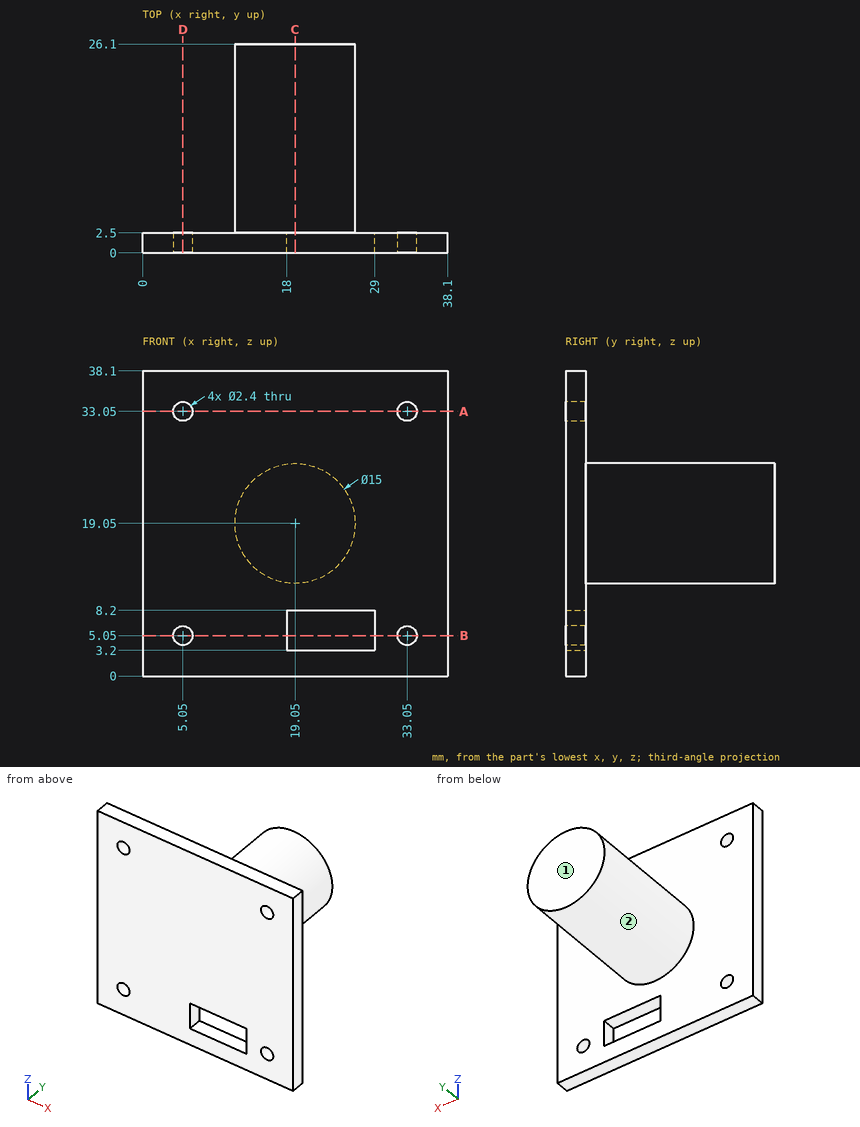
Could you check a few things on this drawing? It's one solid part, dimensions in mm from its lowest x, y, z. A direction names the side the tool comes from. Give positions to 0.01 mm unless a question says otherwise; leave off trailing zeros. Loops run counter-clockwise (first coordinate to the right, second up) from the corner with the lowest first, then second, coordinate; pieces in that order, holes last. Notation, with made-up numbers: (2, -14.75) -> (41, -14.75) arc R16 ccw to (41, 3.25) -> close; hole circle Ø5 at (77, 35). An arc over 180 degrees is marked (long way). Use one line per item in the form item = value. Start each with the question number.
1) For P1, Ø3, axis at x = 14.5, y = 18.5, coming from the +Z side; P2, Ø2, axis at x = 25, y = 1.5, coming from the -Z side; P3, Ø12, axis at y = 10, z = 26, coming from the +X side; P4, Ø1, axis at y = 11.5, z = 16, coming from the +X side, each with a flat end and sliding along its axis, tell me the tip position at first contact or that it passes through.
2) Which directions (+Z, -Z, +X, -X, +Y, -Y) give clear straight access to the entire face, cutting with the end or side of a thin tool? Please do the marked faces 1 and 2.
3) Imagine slicing it at B-B (z = 5.05). Please give me the cut outline in (x, y).
4) Imagine slicing it at C-C (x = 19.05). Please give me the cut outline in (y, z), then the cut area to 3 significant figures.
5) Imagine slicing it at A-A (z = 33.05). Please give me the cut outline in (x, y).
6) Imagine slicing it at D-D (x = 5.05). Please give me the cut outline in (y, z), then the cut area to 4 significant figures.
7) Please list where these lines run through material, in increasing order: line 1 along Z through (x, y) = (5.05, 1.45); line 2 along Y through (x, z) = (17, 9.5).
Check values:
q1.P1 = 25.9
q1.P2 = 0
q1.P3 = 26.49
q1.P4 = 26.1
q2.face_1 = +Z, -Z, +X, -X, +Y
q2.face_2 = +Y
q3.outline = (0, 0) -> (3.85, 0) -> (3.85, 2.5) -> (0, 2.5) -> close; (6.25, 0) -> (18, 0) -> (18, 2.5) -> (6.25, 2.5) -> close; (29, 0) -> (31.85, 0) -> (31.85, 2.5) -> (29, 2.5) -> close; (34.25, 0) -> (38.1, 0) -> (38.1, 2.5) -> (34.25, 2.5) -> close
q4.outline = (0, 0) -> (2.5, 0) -> (2.5, 3.2) -> (0, 3.2) -> close; (0, 8.2) -> (2.5, 8.2) -> (2.5, 11.55) -> (26.1, 11.55) -> (26.1, 26.55) -> (2.5, 26.55) -> (2.5, 38.1) -> (0, 38.1) -> close
q4.area = 437 mm^2
q5.outline = (0, 0) -> (3.85, 0) -> (3.85, 2.5) -> (0, 2.5) -> close; (6.25, 0) -> (31.85, 0) -> (31.85, 2.5) -> (6.25, 2.5) -> close; (34.25, 0) -> (38.1, 0) -> (38.1, 2.5) -> (34.25, 2.5) -> close
q6.outline = (0, 0) -> (2.5, 0) -> (2.5, 3.85) -> (0, 3.85) -> close; (0, 6.25) -> (2.5, 6.25) -> (2.5, 31.85) -> (0, 31.85) -> close; (0, 34.25) -> (2.5, 34.25) -> (2.5, 38.1) -> (0, 38.1) -> close
q6.area = 83.25 mm^2
q7.line_1 = 0 to 3.85, 6.25 to 31.85, 34.25 to 38.1
q7.line_2 = 0 to 2.5
